Verification items for this drawing (mm, ordinates from the low corner). A direction names the side the tool comes from. Give positions to 0.01 mm unless a question says otherwise; leave off trailing zeros. Loops run counter-clockwise (first coordinate to the right, second up) from the corner with the lowest first, then second, coordinate; pieces in that order, holes last. Notation, with made-up numbers: (-32, 86) -> (-16, 86) arc R23 cw to (-16, 106) -> close; hole circle Ø3 at (76.5, 66). An arc over 180 degrees is marked (long way). Answer in a Markdown table with one row per item. Add a question column.
Q1. Section check B-B on z = 0.55. Give the number of separate pieces and of enclosed holes in the cut face, and give its area (3 significant figures).
Q2. Material ranges on probe 1 along X at (y, z) = (11, 2.95); probe 2 along X at (y, z) = (37, 2.7); probe 3 along Y at (x, z) = (15, 2.35) (1 decimal), recorded low to high.
Q3. Set-up check for the marked faces 5 and 6: record each of +Z, -Z, +X, -X, +Y, -Y from which the full face is reachable in a straight line by a thin tool's end or side.
Q4. Release check for a two-part mould opening along X. For the marked faces 1, 2, 3 and 4 record: pulls with the +X half, pulls with the -X half, needs draft (parallel to the pull), parting line crosses it, or undercut.
Q5. Gauge pin test, flat ends, axial feed: P1, Ø1, axis at y = 9.5, z = 2, coming from the +X side; P2, Ø4.5, axis at x = 15.87, y = 35.99, coming from the -Z side; P3, Ø1.6, axis at y = 11, z = 1.5, coming from the -X side. Record the tip position at first contact, or that the pin passes through.
Q6. Section check C-C on y = 14. Enter the section's corners in (x, z) (1 decimal).
Q7. Section check D-D on x = 8.75. Enter the section's corners in (y, z) (1 decimal), and give its area (3 significant figures).
Q8. Section check A-A on y = 35. Enter the section's corners in (x, z) (1 decimal).
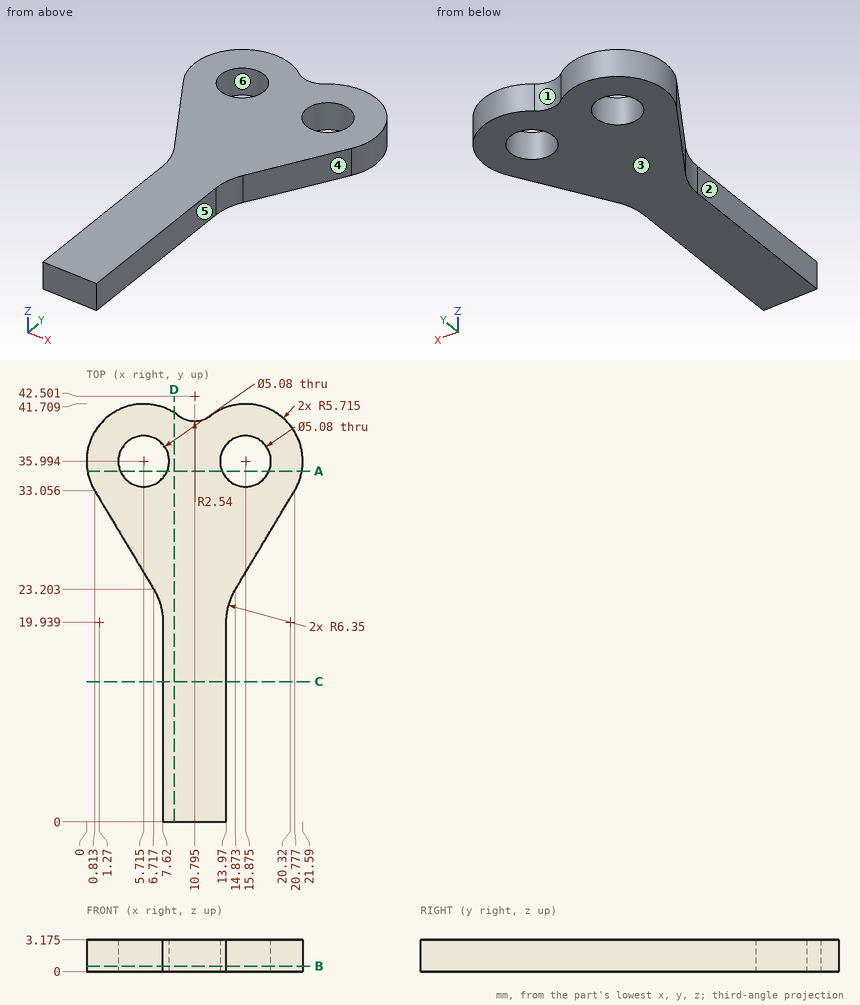
Taken from the geometry:
| question | item | result |
|---|---|---|
| 1 | separate pieces | 1 |
| 1 | enclosed holes | 2 |
| 1 | area | 411 mm² |
| 2 | probe 1 | x = 7.62 to 13.97 |
| 2 | probe 2 | x = 0.09 to 3.38, 8.05 to 13.54, 18.21 to 21.5 |
| 2 | probe 3 | y = 23.4 to 33.6, 38.4 to 41.6 |
| 3 | face 5 | +Z, -Z, +X, -Y |
| 3 | face 6 | +Z, -Z |
| 4 | face 1 | undercut |
| 4 | face 2 | pulls with the -X half |
| 4 | face 3 | needs draft |
| 4 | face 4 | pulls with the +X half |
| 5 | P1 | stops at x = 13.97 |
| 5 | P2 | passes through |
| 5 | P3 | stops at x = 7.62 |
| 6 | outline | (7.6, 0) -> (14, 0) -> (14, 3.2) -> (7.6, 3.2) -> close |
| 7 | outline | (0, 0) -> (40.8, 0) -> (40.8, 3.2) -> (0, 3.2) -> close |
| 7 | area | 130 mm² |
| 8 | outline | (0.1, 0) -> (3.4, 0) -> (3.4, 3.2) -> (0.1, 3.2) -> close; (8.1, 0) -> (13.5, 0) -> (13.5, 3.2) -> (8.1, 3.2) -> close; (18.2, 0) -> (21.5, 0) -> (21.5, 3.2) -> (18.2, 3.2) -> close |
